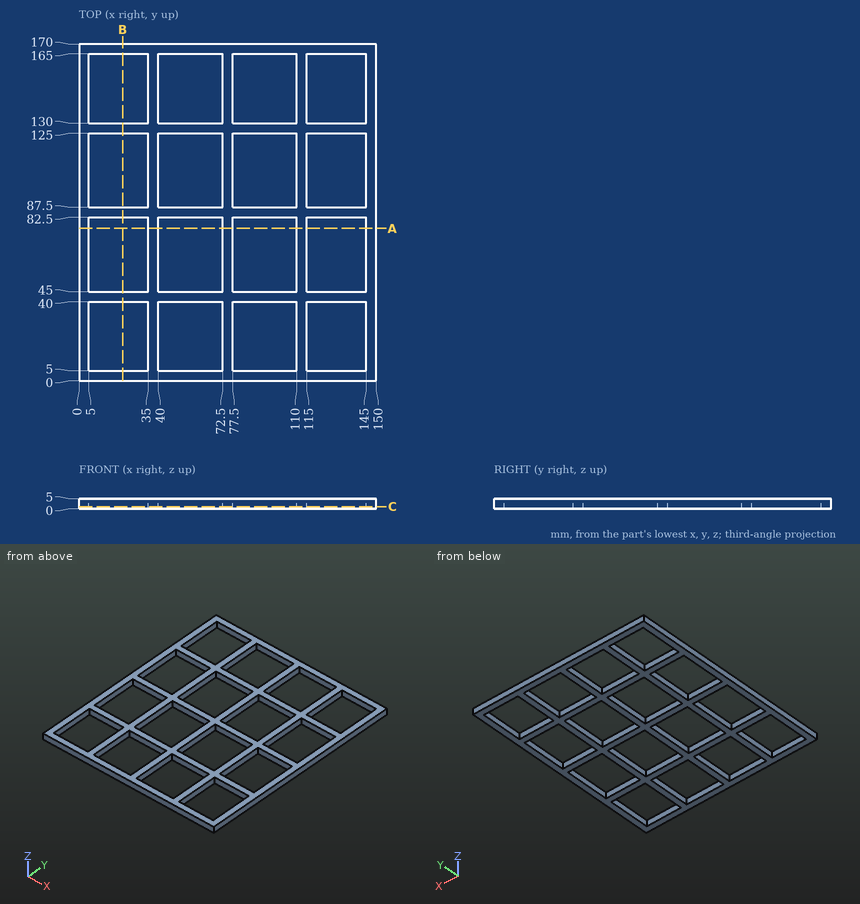
Part print with two shaded views. Sizes in mm from the minimum x, y, z corner. Round coordinates to 2 decimals unless told otherwise and drop trailing zeros. Loops run counter-clockwise (first coordinate to the right, second up) from the corner with the lowest first, then second, coordinate; pieces in that order, holes last. Notation, with made-up numbers: M -7,51 L 44,51 A17 cw 44,67 Z; hole C 58.5,-20 d10. An arc over 180 degrees is marked long. Put each result on its own line as item: value. Start each with the question number.
Item 1: Cut at A-A (y = 77). List the corners of the cut face in (x, z).
Item 2: Cut at B-B (x = 22). List the corners of the cut face in (y, z), then the cut area to 3 significant figures.
Item 3: Cut at C-C (z = 1.05). Give the number of separate pieces and of enclosed holes in the cut face, then the cut area to 4 significant figures.
Item 4: Drill centre lines: line 1 along Y through (x, z) = (131.5, 1.85); line 2 along X through (y, z) = (81, 3.3). Where is each one in solid material? Low to high.
Answer block:
1. outline: M 0,0 L 5,0 L 5,5 L 0,5 Z; M 35,0 L 40,0 L 40,5 L 35,5 Z; M 72.5,0 L 77.5,0 L 77.5,5 L 72.5,5 Z; M 110,0 L 115,0 L 115,5 L 110,5 Z; M 145,0 L 150,0 L 150,5 L 145,5 Z
2. outline: M 0,0 L 5,0 L 5,5 L 0,5 Z; M 40,0 L 45,0 L 45,5 L 40,5 Z; M 82.5,0 L 87.5,0 L 87.5,5 L 82.5,5 Z; M 125,0 L 130,0 L 130,5 L 125,5 Z; M 165,0 L 170,0 L 170,5 L 165,5 Z
2. area: 125 mm2
3. separate pieces: 1
3. enclosed holes: 16
3. area: 7,375 mm2
4. line 1: 0 to 5, 40 to 45, 82.5 to 87.5, 125 to 130, 165 to 170
4. line 2: 0 to 5, 35 to 40, 72.5 to 77.5, 110 to 115, 145 to 150
